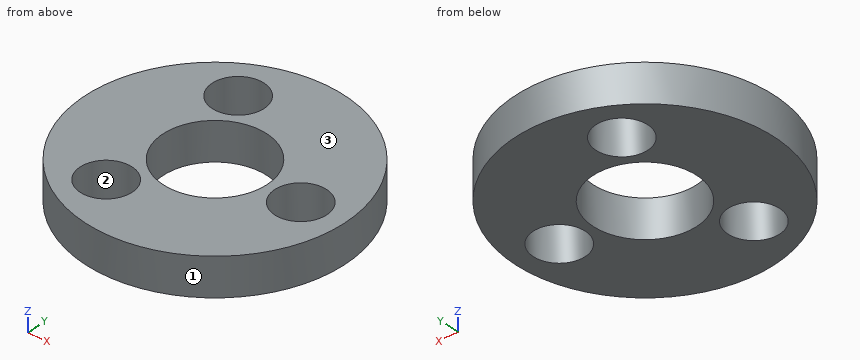
from build123d import *

# Parameters (mm, degrees)
SKETCH_1_R     = 37.5
PAD_1_DEPTH    = 11
SKETCH_2_R     = 15
POCKET_2_DEPTH = 11.001
SKETCH_3_R     = 4.5
POCKET_3_DEPTH = 11.001
SKETCH_4_R     = 4.5
POCKET_4_DEPTH = 11.001
SKETCH_5_R     = 4.5
POCKET_5_DEPTH = 11.001
SKETCH_6_R     = 7.5
POCKET_6_DEPTH = 11.001
SKETCH_7_R     = 7.5
POCKET_7_DEPTH = 11.001
SKETCH_8_R     = 7.5
POCKET_8_DEPTH = 11.001


with BuildPart() as part:
    # Sketch_1 → Pad_1 (new body)
    with BuildSketch(Plane.XY):
        Circle(SKETCH_1_R)
    extrude(amount=PAD_1_DEPTH)

    # Sketch_2 (on Face3 of Pad_1) → Pocket_2 (cut, through all)
    with BuildSketch(Plane.XY.offset(11)):
        Circle(SKETCH_2_R)
    extrude(amount=-POCKET_2_DEPTH, mode=Mode.SUBTRACT)

    # Sketch_3 (on Face3 of Pocket_2) → Pocket_3 (cut, through all)
    with BuildSketch(Plane.XY.offset(11)):
        with Locations((25, 0)):
            Circle(SKETCH_3_R)
    extrude(amount=-POCKET_3_DEPTH, mode=Mode.SUBTRACT)

    # Sketch_4 (on Face3 of Pocket_3) → Pocket_4 (cut, through all)
    with BuildSketch(Plane.XY.offset(11)):
        with Locations((-12.5, 21.65)):
            Circle(SKETCH_4_R)
    extrude(amount=-POCKET_4_DEPTH, mode=Mode.SUBTRACT)

    # Sketch_5 (on Face3 of Pocket_4) → Pocket_5 (cut, through all)
    with BuildSketch(Plane.XY.offset(11)):
        with Locations((-12.5, -21.65)):
            Circle(SKETCH_5_R)
    extrude(amount=-POCKET_5_DEPTH, mode=Mode.SUBTRACT)

    # Sketch_6 (on Face3 of Pocket_5) → Pocket_6 (cut, through all)
    with BuildSketch(Plane.XY.offset(11)):
        with Locations((25, 0)):
            Circle(SKETCH_6_R)
    extrude(amount=-POCKET_6_DEPTH, mode=Mode.SUBTRACT)

    # Sketch_7 (on Face3 of Pocket_6) → Pocket_7 (cut, through all)
    with BuildSketch(Plane.XY.offset(11)):
        with Locations((-12.5, 21.65)):
            Circle(SKETCH_7_R)
    extrude(amount=-POCKET_7_DEPTH, mode=Mode.SUBTRACT)

    # Sketch_8 (on Face3 of Pocket_7) → Pocket_8 (cut, through all)
    with BuildSketch(Plane.XY.offset(11)):
        with Locations((-12.5, -21.65)):
            Circle(SKETCH_8_R)
    extrude(amount=-POCKET_8_DEPTH, mode=Mode.SUBTRACT)


solid = part.part
Geometry check sheet. Reference: the model listing, model coordinates, mm. Face numbers are marked on the shaded views. Give positions to 0.01 mm unless a question says otherwise; leave off trailing zeros. Order: outer loops, then holes, each group sorted by start corner. A loop starts at its lowest first (then second) coordinate and runs counter-clockwise, first axis right, second up. Notation, with made-up numbers: M 33.5,-29.5 L 83.5,-29.5 A33 ccw 83.5,-0.5 Z; hole C 85,52 d1. An arc over 180 degrees is marked long. Use a Markdown table: item, result.
Item 1: Section check B-B (y = 0). Record the cut outline in (x, z).
Answers follow:
| item | result |
|---|---|
| outline | M -37.5,0 L -15,0 L -15,11 L -37.5,11 Z; M 15,0 L 17.5,0 L 17.5,11 L 15,11 Z; M 32.5,0 L 37.5,0 L 37.5,11 L 32.5,11 Z |
Item 2: Section check D-D (z = 1.25). Record the cut outline in (x, y), and give its area (3 significant figures).
Answers follow:
| item | result |
|---|---|
| outline | C 0,0 d75; hole C -12.5,-21.65 d15; hole C -12.5,21.65 d15; hole C 0,0 d30; hole C 25,0 d15 |
| area | 3,180 mm2 |
Item 3: Material ranges on line 1 along Y through (x, z) = (0, 7); line 2 along X through (y, z) = (0.5, 8.5); line 3 along Y through (x, z) = (-12.5, 4.5), recorded low to high.
Answers follow:
| item | result |
|---|---|
| line 1 | y = -37.5 to -15, 15 to 37.5 |
| line 2 | x = -37.5 to -14.99, 14.99 to 17.52, 32.48 to 37.5 |
| line 3 | y = -35.36 to -29.15, -14.15 to -8.29, 8.29 to 14.15, 29.15 to 35.36 |
Item 4: Section check A-A (x = 0). Record the cut outline in (y, z), and give its area (3 significant figures).
Answers follow:
| item | result |
|---|---|
| outline | M -37.5,0 L -15,0 L -15,11 L -37.5,11 Z; M 15,0 L 37.5,0 L 37.5,11 L 15,11 Z |
| area | 495 mm2 |
Item 5: Draft check along X on the marked faces 1, 2 and 3. Enter one of: +X half, -X half, draft (parallel to the pull), parting line (faces both ways), or undercut.
Answers follow:
| item | result |
|---|---|
| face 1 | parting line |
| face 2 | undercut |
| face 3 | draft |
Item 6: Depth check by flat-ended pin: P1, Ø19.5, axis at x = 25, y = 0, coming from the -Z side; P2, Ø24, axis at x = 0, y = 0, coming from the -Z side; P3, Ø2, axis at x = -1.5, z = 3.5, coming from the +Y side; P4, Ø1.5, axis at x = -4.5, z = 7.5, coming from the -Y side. Enter the tip coordinate at first touch or a pass-through.
Answers follow:
| item | result |
|---|---|
| P1 | stops at z = 0 |
| P2 | passes through |
| P3 | stops at y = 37.5 |
| P4 | stops at y = -37.31 |
Item 7: Section check C-C (y = 16). Record the cut outline in (x, z), and give its area (3 significant figures).
Answers follow:
| item | result |
|---|---|
| outline | M -33.92,0 L -17.43,0 L -17.43,11 L -33.92,11 Z; M -7.57,0 L 33.92,0 L 33.92,11 L -7.57,11 Z |
| area | 638 mm2 |
